Autodesk Fusion 360 part; units mm, degrees
sketch "Name Sign Support" plane through (0, 0, 0) normal (1, 0, 0) x (0, 1, 0) in component "Name Sign Support (1)"
  line L0 (-0.0158, 97.2466) -> (23.9842, 87.4035)
  line L1 (23.9842, 142.8255) -> (-0.0158, 152.6686)
  line L2 (-0.0158, 152.6686) -> (-0.0158, 97.2466)
  line L3 (23.9842, 142.8255) -> (23.9842, 87.4035)
  dimension "d18" = 67.7
  dimension "d8" = 24
  dimension "d9" = 55.422
extrude "Extrude2" add sketch "Name Sign Support" along normal blind 12 in component "Name Sign Support (1)"
component "Name Sign Support Right" placed x (1, 0, 0) y (0, 1, 0) z (0, 0, 1) at (0, 0, 0)
component "Name Sign Support (1)" placed x (1, 0, 0) y (0, 1, 0) z (0, 0, 1) at (0, 0, 0) in component "Name Sign Support Right"
equation "d19 = pineThickness"
equation "pineThickness = 12 mm"
For this review, take the finished solid that the model builds, in its own axes (mm). Give positions to 0.01 mm unless a question says otherwise; leave off trailing zeros. Loops run counter-clockwise (first coordinate to the right, second up) from the corner with the lowest first, then second, coordinate; pieces in that order, holes last. Notation, with made-up numbers: M 59,-21 L 99,-21 A29 cw 99,7 Z; hole C -15,3.5 d9. An arc over 180 degrees is marked long. Answer as a JSON object with one key per item and string values. Group by question number.
Q1. Add section A-A on x = 9.5. Give the boundary of the cut face in (y, z).
Q2. Add section B-B on y = 20. Give the boundary of the cut face in (x, z).
Q3. For probe 1 along Z at (x, y) = (4, 16.75); probe 2 along Z at (x, y) = (6.75, 9.5); probe 3 along Y at (x, z) = (3.5, 144), list the stretches that pass through material, from the lowest coordinate up. Write a range as [from, to].
Q4. Insertion check: P1, Ø1.5, axis at x = 7.5, y = 13.5, coming from the -Z side; P2, Ø10, axis at y = 15.5, z = 99, coming from the -X side; P3, Ø5, axis at x = 1.5, y = 11.5, coming from the -Z side; P4, Ø6, axis at x = 5.5, y = 12.5, coming from the -Z side. Each pin has a flat end and moves straight along its axis. Give the tip position at first contact, or say it passes through.
Checked values:
{
 "1": {"outline": "M -0.02,97.25 L 23.98,87.4 L 23.98,142.83 L -0.02,152.67 Z"},
 "2": {"outline": "M 0,89.04 L 12,89.04 L 12,144.46 L 0,144.46 Z"},
 "3": {"probe 1": "[90.37, 145.79]", "probe 2": "[93.34, 148.77]", "probe 3": "[-0.02, 21.12]"},
 "4": {"P1": "z = 91.4", "P2": "x = 0", "P3": "z = 91.5", "P4": "z = 90.88"}
}
